from build123d import *

# Parameters (mm, degrees)
SKETCH1_W           = 11.4
SKETCH1_H           = 4.75
BOSS_EXTRUDE1_DEPTH = 0.5
BOSS_EXTRUDE2_DEPTH = 3.5
BOSS_EXTRUDE3_DEPTH = 0.35
FILLET1_R           = 0.1


with BuildPart() as part:
    # Sketch1 → Boss-Extrude1 (new body)
    with BuildSketch(Plane(origin=(0, 0, 0), x_dir=(1, 0, 0), z_dir=(0, 1, 0))):
        Rectangle(SKETCH1_W, SKETCH1_H)
    extrude(amount=BOSS_EXTRUDE1_DEPTH)

    # Sketch2 → Boss-Extrude2 (add)
    with BuildSketch(Plane(origin=(0, 0.5, 0), x_dir=(1, 0, 0), z_dir=(0, 1, 0))):
        with BuildLine():
            Line((-3.15, 1.8), (3.15, 1.8))
            ThreePointArc((3.15, 1.8), (4.95, 0), (3.15, -1.8))
            Line((3.15, -1.8), (-3.15, -1.8))
            ThreePointArc((-3.15, -1.8), (-4.95, 0), (-3.15, 1.8))
        make_face()
    extrude(amount=BOSS_EXTRUDE2_DEPTH)

    # Sketch2_3 → Boss-Extrude3 (add)
    with BuildSketch(Plane(origin=(0, 0.5, 0), x_dir=(1, 0, 0), z_dir=(0, 1, 0))):
        with BuildLine():
            Line((-3.15, 2.15), (3.15, 2.15))
            ThreePointArc((3.15, 2.15), (5.3, 0), (3.15, -2.15))
            Line((3.15, -2.15), (-3.15, -2.15))
            ThreePointArc((-3.15, -2.15), (-5.3, 0), (-3.15, 2.15))
        make_face()
        with BuildLine():
            Line((-3.15, 1.8), (3.15, 1.8))
            ThreePointArc((3.15, 1.8), (4.95, 0), (3.15, -1.8))
            Line((3.15, -1.8), (-3.15, -1.8))
            ThreePointArc((-3.15, -1.8), (-4.95, 0), (-3.15, 1.8))
        make_face(mode=Mode.SUBTRACT)
    extrude(amount=BOSS_EXTRUDE3_DEPTH)

    # Fillet1
    fillet1_edges = [part.edges().sort_by_distance(p)[0] for p in [
        (0, 4, -1.8),
        (0, 4, 1.8),
        (4.95, 4, 0),
        (-4.95, 4, 0),
        (-4.95, 0.85, 0),
        (0, 0.85, 1.8),
        (4.95, 0.85, 0),
        (0, 0.85, -1.8),
    ]]
    fillet(fillet1_edges, radius=FILLET1_R)


solid = part.part
Source: CAD feature listing. Evaluate the final solid. Frame: model axes, mm. A direction names the side the tool comes from. Give positions to 0.01 mm unless a question says otherwise; leave off trailing zeros. Loops run counter-clockwise (first coordinate to the right, second up) from the corner with the lowest first, then second, coordinate; pieces in that order, holes last. Notation, with made-up numbers: (-11.75, 26) -> (2.25, 26) arc R20 cw to (2.25, 56) -> close; hole circle Ø11 at (-1, 63.5). An arc over 180 degrees is marked (long way). Use a Markdown table: item, result. Add a question column.
1) Section query B-B, the plane x = 3. Return the cut outline in (y, z) (3 decimals), then the cut area to 3 significant figures.
2) Section query C-C, the plane y = 2.05. Return the cut outline in (x, z).
3) Section query A-A, the plane z = 0. Return the cut outline in (x, y), then the cut area to 3 significant figures.
4) Line query: line 1 along Y through (x, z) = (-2.5, -2.1); line 2 along Z through (x, y) = (-1.25, 2.7); line 3 along X through (y, z) = (0.6, 0). Output: solid intervals per line, ascending. Write a range as [from, to].
5) First-contact query: pin 1 (0.9 mm diameter, centred on x = 0, y = 1.5, fed in from -Z); pin 2 (1.5 mm diameter, centred on x = 3.5, y = 1, fed in from +Z) (3 decimals). Flat tips, straight axial feed; report the tip coordinate or a pass-through.
6) Reachability of faces 1 (the face through (0, 2, 1.8)), 2 (the face through (5.3, 0.7, 0)), 3 (the face through (0, 2, -1.8)), 4 (the face through (-5.3, 0.7, 0)) from +Z, -Z, +X, -X, +Y, -Y: full face, straight path, thin tool, end or side. Return the list, or none.
Numbers:
| question | item | result |
|---|---|---|
| 1 | outline | (0, -2.375) -> (0.5, -2.375) -> (0.5, -2.15) -> (0.85, -2.15) -> (0.85, -1.9) arc R0.1 cw to (0.95, -1.8) -> (3.9, -1.8) arc R0.1 ccw to (4, -1.7) -> (4, 1.7) arc R0.1 ccw to (3.9, 1.8) -> (0.95, 1.8) arc R0.1 cw to (0.85, 1.9) -> (0.85, 2.15) -> (0.5, 2.15) -> (0.5, 2.375) -> (0, 2.375) -> close |
| 1 | area | 15.2 mm2 |
| 2 | outline | (-3.15, -1.8) -> (3.15, -1.8) arc R1.8 ccw to (3.15, 1.8) -> (-3.15, 1.8) arc R1.8 ccw to start |
| 3 | outline | (-5.7, 0) -> (5.7, 0) -> (5.7, 0.5) -> (5.3, 0.5) -> (5.3, 0.85) -> (5.05, 0.85) arc R0.1 cw to (4.95, 0.95) -> (4.95, 3.9) arc R0.1 ccw to (4.85, 4) -> (-4.85, 4) arc R0.1 ccw to (-4.95, 3.9) -> (-4.95, 0.95) arc R0.1 cw to (-5.05, 0.85) -> (-5.3, 0.85) -> (-5.3, 0.5) -> (-5.7, 0.5) -> close |
| 3 | area | 40.6 mm2 |
| 4 | line 1 | y = [0, 0.85] |
| 4 | line 2 | z = [-1.8, 1.8] |
| 4 | line 3 | x = [-5.3, 5.3] |
| 5 | pin 1 | stops at z = -1.8 |
| 5 | pin 2 | stops at z = 2.375 |
| 6 | face 1 | +Z, +X, -X, +Y |
| 6 | face 2 | +X, +Y |
| 6 | face 3 | -Z, +X, -X, +Y |
| 6 | face 4 | -X, +Y |
